Study the drawing (mm; zero at the part's minimum x, y, z) and answer. A direction names the side the tool comes from. Coordinates: 2 decimals unless noted, no trailing zeros. Order: outer loops, then holes, each group sorted by start corner. A loop starts at its lowest first (then second) coordinate and runs counter-clockwise, first axis right, second up. Notation, with made-up numbers: (20.5, -11) -> (37.5, -11) arc R11 ccw to (37.5, -2) -> close; hole circle Ø11 at (10, -36). An arc over 180 degrees is marked (long way). Answer in a Markdown table with one row per item. Add a question column.
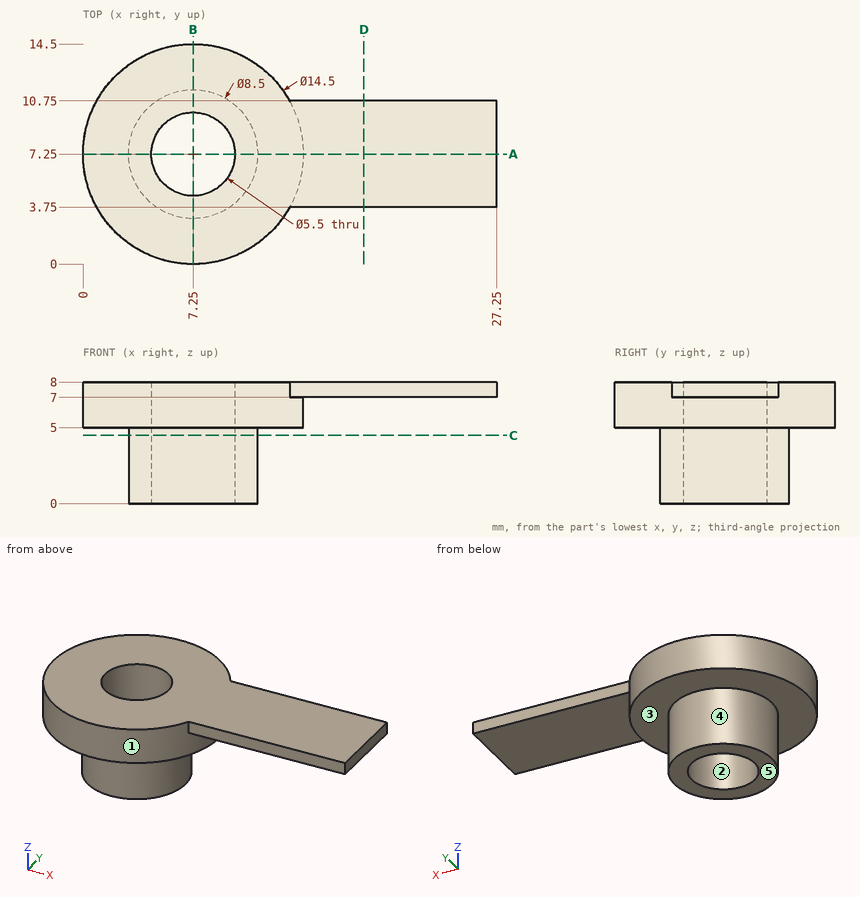
Q1. A cutting plane is placed at D-D (x = 18.5). Determine the outline of the cut face in (y, z), then the cut area to 3 significant figures.
Q2. A cutting plane is placed at B-B (x = 7.25). Determine the outline of the cut face in (y, z).
Q3. Straight lines are drawn through the part: line 1 (Y direction, x = 7.25, z = 5.75); line 2 (Y direction, x = 7.25, z = 4.75); line 3 (Z direction, x = 25, y = 6.25). For each, find the intervals that lie inside material, in ascending order.
Q4. A cutting plane is placed at C-C (z = 4.5). Determine the outline of the cut face in (x, y), then the cut area to 3 significant figures.
Q5. Given pin 1 (2 mm diameter, centred on y = 9.5, z = 1, fed in from -X); pin 2 (3.5 mm diameter, centred on x = 20, y = 7.5, fed in from -Z); pin 3 (2 mm diameter, centred on y = 12, z = 1.5, fed in from -X), each flat-ended and moving along its own axis, determine where each tip first touches the part or whether it passes through.
Q6. For the marked faces 4 and 5, determine the directions among +Z, -Z, +X, -X, +Y, -Y from which every point of the face is accessible in a straight line to the end or side of a thin tool.
Q7. Determine the mould class of the marked faces 1, 2 and 3 for opening direction X: +X half, -X half, draft (parallel to the pull), parting line (faces both ways), or undercut.
Q8. A cutting plane is placed at A-A (y = 7.25). Determine the outline of the cut face in (x, z), then the cut area to 4 significant figures.
Returned:
| question | item | result |
|---|---|---|
| 1 | outline | (3.75, 7) -> (10.75, 7) -> (10.75, 8) -> (3.75, 8) -> close |
| 1 | area | 7.00 mm² |
| 2 | outline | (0, 5) -> (3, 5) -> (3, 0) -> (4.5, 0) -> (4.5, 8) -> (0, 8) -> close; (10, 0) -> (11.5, 0) -> (11.5, 5) -> (14.5, 5) -> (14.5, 8) -> (10, 8) -> close |
| 3 | line 1 | y = 0 to 4.5, 10 to 14.5 |
| 3 | line 2 | y = 3 to 4.5, 10 to 11.5 |
| 3 | line 3 | z = 7 to 8 |
| 4 | outline | circle Ø8.5 at (7.25, 7.25); hole circle Ø5.5 at (7.25, 7.25) |
| 4 | area | 33.0 mm² |
| 5 | pin 1 | stops at x = 3.19 |
| 5 | pin 2 | stops at z = 7 |
| 5 | pin 3 | stops at x = 5.25 |
| 6 | face 4 | -Z |
| 6 | face 5 | -Z, +X, -X, +Y, -Y |
| 7 | face 1 | parting line |
| 7 | face 2 | undercut |
| 7 | face 3 | draft |
| 8 | outline | (0, 5) -> (3, 5) -> (3, 0) -> (4.5, 0) -> (4.5, 8) -> (0, 8) -> close; (10, 0) -> (11.5, 0) -> (11.5, 5) -> (14.5, 5) -> (14.5, 7) -> (27.25, 7) -> (27.25, 8) -> (10, 8) -> close |
| 8 | area | 54.75 mm² |
